Geometry: see drawing. Coordinates: mm, zero at the bounding-box minimum. A direction names the side the tool comes from. Round coordinates to 2 decimals unless told otherwise and drop trailing zeros. Write each loop counter-clockwise with the first axis right and the second up, starting at its lowest first coordinate (ties: lowest second). Pieces come first, ordered by that corner, then holes. Notation, with made-up numbers: (75, -2.5) - (97, -2.5) arc R20 ccw to (97, 32.5) - close; hole circle Ø2 at (17.25, 3). An arc over 180 degrees is marked (long way). One line per item, written item: value. Start each with the question number.
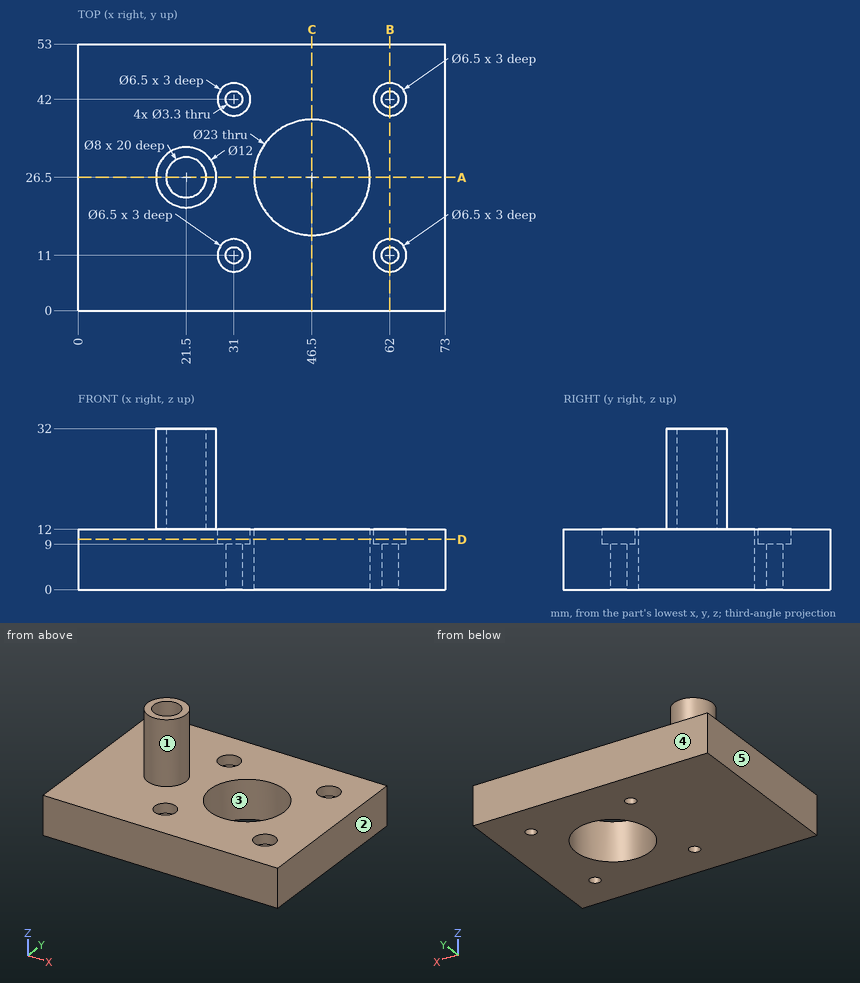
Q1. Cut plane B-B, the plane x = 62. Output: boundary loops of the cut face in (y, z), and give its area (3 significant figures).
Q2. Cut plane A-A, the plane y = 26.5. Output: boundary loops of the cut face in (x, z).
Q3. Access query for the marked faces 1 and 2. Directions: +Z, -Z, +X, -X, +Y, -Y. A direction counts if a zero-diameter tool reaches every point of the face in a straight line with its end or side. Return the directions, or none.
Q4. Pull-direction query (X, two-part tool) for the marked faces 3, 4 and 5; classes: pulls with the +X half, pulls with the -X half, needs draft (parallel to the pull), parting line crosses it, or undercut.
Q5. Material intervals for probe 1 along Y at (x, z) = (31, 9.65); probe 2 along Y at (x, z) = (31, 2); probe 3 along Y at (x, z) = (46.5, 8.5), sorted ascending. Write a range as from..to.
Q6. Cut plane D-D, the plane z = 10. Output: boundary loops of the cut face in (x, y).
Q7. Cut plane C-C, the plane x = 46.5. Output: boundary loops of the cut face in (y, z), and give its area (3 significant figures).
Q8. Contact query for flat-ended pins moving along their axis: pin 1 Ø2 at (x, y) = (31, 11) entering from +Z; pin 2 Ø2 at (y, z) = (32.5, 24) entering from +X; pin 3 Ø16 at (x, y) = (40.5, 20.5) entering from +Z; pin 4 Ø5 at (x, y) = (61.5, 11) entering from +Z. Output: stop coordinate, or through.
A:
1. outline: (0, 0) - (9.35, 0) - (9.35, 9) - (7.75, 9) - (7.75, 12) - (0, 12) - close; (12.65, 0) - (40.35, 0) - (40.35, 9) - (38.75, 9) - (38.75, 12) - (14.25, 12) - (14.25, 9) - (12.65, 9) - close; (43.65, 0) - (53, 0) - (53, 12) - (45.25, 12) - (45.25, 9) - (43.65, 9) - close
1. area: 538 mm²
2. outline: (0, 0) - (35, 0) - (35, 12) - (27.5, 12) - (27.5, 32) - (25.5, 32) - (25.5, 12) - (17.5, 12) - (17.5, 32) - (15.5, 32) - (15.5, 12) - (0, 12) - close; (58, 0) - (73, 0) - (73, 12) - (58, 12) - close
3. face 1: +Z
3. face 2: +Z, -Z, +X, +Y, -Y
4. face 3: undercut
4. face 4: needs draft
4. face 5: pulls with the -X half
5. probe 1: y = 0..7.75, 14.25..38.75, 45.25..53
5. probe 2: y = 0..9.35, 12.65..40.35, 43.65..53
5. probe 3: y = 0..15, 38..53
6. outline: (0, 0) - (73, 0) - (73, 53) - (0, 53) - close; hole circle Ø6.5 at (31, 11); hole circle Ø6.5 at (31, 42); hole circle Ø23 at (46.5, 26.5); hole circle Ø6.5 at (62, 11); hole circle Ø6.5 at (62, 42)
7. outline: (0, 0) - (15, 0) - (15, 12) - (0, 12) - close; (38, 0) - (53, 0) - (53, 12) - (38, 12) - close
7. area: 360 mm²
8. pin 1: passes through
8. pin 2: stops at x = 24.82
8. pin 3: stops at z = 12
8. pin 4: stops at z = 9
